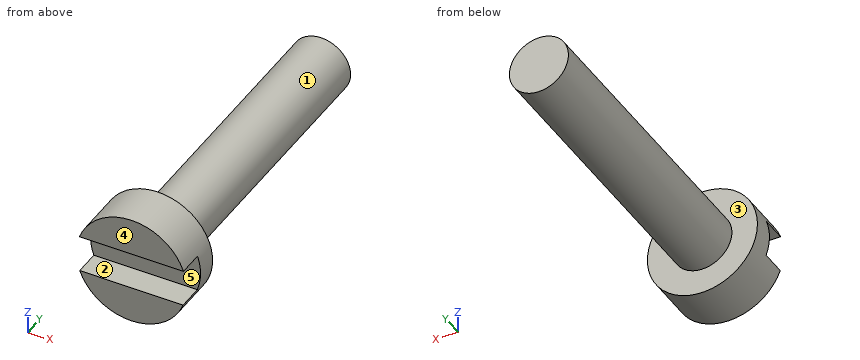
Autodesk Inventor part; units mm, degrees
ref_plane "YZ Plane" through (0, 0, 0) normal (1, 0, 0) x (0, 1, 0)
ref_plane "XZ Plane" through (0, 0, 0) normal (0, 1, 0) x (-1, 0, 0)
ref_plane "XY Plane" through (0, 0, 0) normal (0, 0, 1) x (1, 0, 0)
sketch "Esboço1" plane through (0, 0, 0) normal (0, 1, 0) x (-1, 0, 0)
  circle A0 centre (0, 0) radius 2.8
  dimension "d0" = 5.6
extrude "Extrusão1" add sketch "Esboço1" along normal blind 2.4
sketch "Esboço2" plane through (0, 0, 0) normal (1, 0, 0) x (0, 1, 0)
  line L0 (0, 0.9185) -> (1.2961, 0.9185)
  line L1 (1.2961, 0.9185) -> (1.2961, -0.9611)
  line L2 (1.2961, -0.9611) -> (0, -0.9611)
  line L3 (0, -0.9611) -> (0, 0.9185)
  point P0 (0, 0)
extrude "Extrusão2" cut sketch "Esboço2" along normal through all both and the other way through all
sketch "Esboço3" plane through (0, 2.4, 0) normal (0, 1, 0) x (1, 0, 0)
  circle A0 centre (0, 0) radius 2.8
  circle A1 centre (0, 0) radius 1.5
  dimension "d5" = 3
extrude "Extrusão3" add sketch "Esboço3" along normal blind 15 contours A1
thread "Rosca1"
properties part number "AA-Parafuso-M3-30"
Can you work these out from the model? Positions are in its coordinate system, mm. Face numbers are marked on the shaded views. A direction names the side the tool comes from. Give positions to 0.01 mm unless a question says otherwise; leave off trailing zeros. Loops run counter-clockwise (first coordinate to the right, second up) from the corner with the lowest first, then second, coordinate; pieces in that order, holes last. Notation, with made-up numbers: M 44.25,81 L 94.25,81 A22 ccw 94.25,98 Z; hole C 13.25,-24.5 d1. An arc over 180 degrees is marked long. One line per item, written item: value. Start each with the question number.
1) If we section it at C-C, the plane y = 13.75: Write out the boundary of the cut face in (x, z), and give its area (3 significant figures).
2) If we section it at B-B, the plane z = 0: Write out the boundary of the cut face in (x, y), and give its area (3 significant figures).
3) Thinking about a two-plate mould opening in Z: for the marked faces 1, 2 and 3, which applies, +Z half, -Z half, draft (parallel to the pull), parting line (faces both ways), or undercut?
4) If we section it at A-A, the plane x = 0: Write out the boundary of the cut face in (y, z), and give its area (3 significant figures).
5) If we section it at D-D, the plane z = 1.2: Write out the boundary of the cut face in (x, y).
6) On a 3-axis mill with a long thin cutter (end or side, diameter ignored), from which of +Z, -Z, +X, -X, +Y, -Y can I reach the whole of each face in a straight line? I mean the marked faces 4 and 5. Say none if no direction works.
7) If I drill on line 1 (Y direction, x = 2.45, z = 0.7); line 2 (Z direction, x = -0.1, y = 15.5); line 3 (Y direction, x = -1.1, z = -2.3), over which ranges is the centre line in solid material (lowest first)? Write a range as [from, to].
8) I'm going to push flat-ended pins straight in: pin 1 (3 mm diameter, centred on x = -1.5, y = 13, fed in from +Z); pin 2 (1.4 mm diameter, centred on x = -1.5, y = 0.5, fed in from -Z); pin 3 (1.5 mm diameter, centred on x = -1, y = 14, fed in from -Z). Where does each tip first touch, or does it pass through?
Completed:
1. outline: C 0,0 d3
1. area: 7.07 mm^2
2. outline: M -2.8,1.3 L 2.8,1.3 L 2.8,2.4 L 1.5,2.4 L 1.5,17.4 L -1.5,17.4 L -1.5,2.4 L -2.8,2.4 Z
2. area: 51.2 mm^2
3. face 1: parting line
3. face 2: undercut
3. face 3: draft
4. outline: M 0,-2.8 L 2.4,-2.8 L 2.4,-1.5 L 17.4,-1.5 L 17.4,1.5 L 2.4,1.5 L 2.4,2.8 L 0,2.8 L 0,0.92 L 1.3,0.92 L 1.3,-0.96 L 0,-0.96 Z
4. area: 56.0 mm^2
5. outline: M -2.53,0 L 2.53,0 L 2.53,2.4 L 0.9,2.4 L 0.9,17.4 L -0.9,17.4 L -0.9,2.4 L -2.53,2.4 Z
6. face 4: +Z, -Z, +X, -X, -Y
6. face 5: +X, -X, -Y
7. line 1: y = [1.3, 2.4]
7. line 2: z = [-1.5, 1.5]
7. line 3: y = [0, 2.4]
8. pin 1: stops at z = 1.5
8. pin 2: stops at z = -2.68
8. pin 3: stops at z = -1.48
